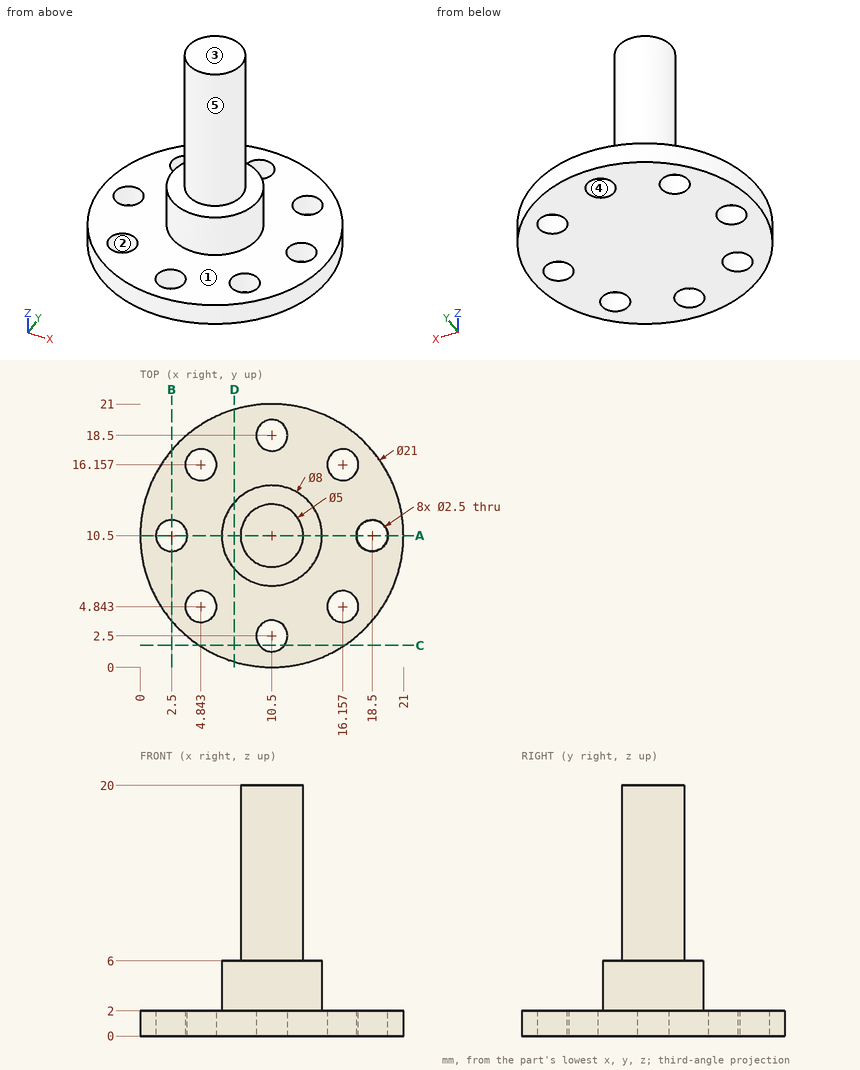
Here's the drawing with two shaded views (mm, measured from the low corner). I have some questions. A direction names the side the tool comes from. Round coordinates to 2 decimals unless told otherwise and drop trailing zeros. Loops run counter-clockwise (first coordinate to the right, second up) from the corner with the lowest first, then second, coordinate; pieces in that order, holes last.
Item 1: Will these pins go through, and if not, where does the flat tip stop? pin 1 Ø12 at (x, z) = (10.5, 16.5) entering from +Y; pin 2 Ø1 at (x, z) = (11.5, 3) entering from -Y; pin 3 Ø4 at (x, y) = (10.5, 18.5) entering from +Z.
Item 2: Please list where these lines run through material, in increasing order: L1, parallel to Y at x = 10.5, z = 0.8; L2, parallel to Z at x = 5.75, y = 12.5; L3, parallel to Z at x = 13.5, y = 11.
Item 3: Suppose I cut it at C-C, the plane y = 1.75. Write out the boundary of the cut face in (x, z), then the cut area to 3 significant figures.
Item 4: Suppose I cut it at A-A, the plane y = 10.5. Write out the boundary of the cut face in (x, z).
Item 5: Suppose I cut it at D-D, the plane x = 7.5. Write out the boundary of the cut face in (y, z).
Item 6: If we mould it in two halves opening along X, with no side actions, what happens to the marked faces 3, 4 and 5? For each: +X half, -X half, draft (parallel to the pull), parting line (faces both ways), or undercut.
Item 7: Suppose I cut it at B-B, the plane x = 2.5. Write out the boundary of the cut face in (y, z).
Item 8: Which directions (+Z, -Z, +X, -X, +Y, -Y) give clear straight access to the entire face, cutting with the end or side of a thin tool? Please do the marked faces 1 and 2.
Reported:
1. pin 1: stops at y = 13
1. pin 2: stops at y = 6.53
1. pin 3: stops at z = 2
2. L1: y = 0 to 1.25, 3.75 to 17.25, 19.75 to 21
2. L2: z = 0 to 2
2. L3: z = 0 to 6
3. outline: (4.7, 0) - (9.5, 0) - (9.5, 2) - (4.7, 2) - close; (11.5, 0) - (16.3, 0) - (16.3, 2) - (11.5, 2) - close
3. area: 19.2 mm2
4. outline: (0, 0) - (1.25, 0) - (1.25, 2) - (0, 2) - close; (3.75, 0) - (17.25, 0) - (17.25, 2) - (14.5, 2) - (14.5, 6) - (13, 6) - (13, 20) - (8, 20) - (8, 6) - (6.5, 6) - (6.5, 2) - (3.75, 2) - close; (19.75, 0) - (21, 0) - (21, 2) - (19.75, 2) - close
5. outline: (0.44, 0) - (20.56, 0) - (20.56, 2) - (13.15, 2) - (13.15, 6) - (7.85, 6) - (7.85, 2) - (0.44, 2) - close
6. face 3: draft
6. face 4: undercut
6. face 5: parting line
7. outline: (3.7, 0) - (9.25, 0) - (9.25, 2) - (3.7, 2) - close; (11.75, 0) - (17.3, 0) - (17.3, 2) - (11.75, 2) - close
8. face 1: +Z
8. face 2: +Z, -Z
